Can you work these out from the model? Positions are in its coordinate system, mm. A direction names the side the tool comes from. Coordinates: 2 decimals unless noted, no trailing zeros. Write each loop counter-clockwise with the first axis right and the second up, starting at its lowest first coordinate (ties: lowest second). Pieces come first, ordered by that corner, then holes. Notation, with made-up numbers: (-38.5, 30) - (-4.5, 30) arc R26 cw to (-4.5, 61) - close; hole circle Ø2 at (81, 72). An arc over 180 degrees is marked (long way). Use one line per item in the form item = value. Start each with the question number.
(1) If I drill on probe 1 along Y at (x, z) = (4, 0.2); probe 2 along Y at (x, z) = (21, 1); probe 3 along X at (y, z) = (-40, 1), over which ranges is the centre line in solid material (lowest first)? Write a range as from..to.
(2) If we section it at A-A on x = 12: Please give me the cut outline in (y, z).
(3) If we section it at B-B on z = 0.5: Please give me the cut outline in (x, y).
(4) For pin 1 Ø0.7 at (y, z) = (8, 1.5) entering from +X, with a flat end and sliding along its axis, tell me the tip position at first contact or that it passes through.
(5) On a 3-axis mill with a long thin cutter (end or side, diameter ignored), from which of +Z, -Z, +X, -X, +Y, -Y can I reach the whole of each face in a straight line? I mean faces 4 (the face through (11, 5.879, 2)), 5 (the face through (1, -48, 1)). Say none if no direction works.
(6) Thinking about a two-plate mould opening in Y: for faces 1 (the face through (-0.5, -41, 2)), 2 (the face through (0, 45, 1)), 3 (the face through (-21.64, -47.1, 1.52)), which applies, pulls with the +Y half, pulls with the -Y half, needs draft (parallel to the pull), parting line crosses it, or undercut?
```python
from build123d import *

# Parameters (mm, degrees)
CROQUIS1_W              = 45
CROQUIS1_H              = 93
SALIENTE_EXTRUIR1_DEPTH = 3
CROQUIS2_W              = 23
CROQUIS2_H              = 3.3
CORTAR_EXTRUIR1_DEPTH   = 3
CROQUIS3_W              = 23
CROQUIS3_H              = 3.3
CORTAR_EXTRUIR2_DEPTH   = 3
REDONDEO1_R             = 3
REDONDEO2_R             = 0.5


with BuildPart() as part:
    # Croquis1 → Saliente-Extruir1 (new body)
    with BuildSketch(Plane.XY):
        with Locations((0, -1.5)):
            Rectangle(CROQUIS1_W, CROQUIS1_H)
    extrude(amount=SALIENTE_EXTRUIR1_DEPTH)

    # Croquis2 → Cortar-Extruir1 (cut)
    with BuildSketch(Plane.XY.offset(3)):
        with Locations((11, 7.529451896)):
            Rectangle(CROQUIS2_W, CROQUIS2_H)
    extrude(amount=-CORTAR_EXTRUIR1_DEPTH, mode=Mode.SUBTRACT)

    # Croquis3 → Cortar-Extruir2 (cut)
    with BuildSketch(Plane.XY.offset(3)):
        with Locations((11, -41.35)):
            Rectangle(CROQUIS3_W, CROQUIS3_H)
    extrude(amount=-CORTAR_EXTRUIR2_DEPTH, mode=Mode.SUBTRACT)

    # Redondeo1
    redondeo1_edges = [part.edges().sort_by_distance(p)[0] for p in [
        (-22.5, 45, 1.5),
        (-22.5, -48, 1.5),
        (22.5, 45, 1.5),
    ]]
    fillet(redondeo1_edges, radius=REDONDEO1_R)

    # Redondeo2
    redondeo2_edges = [part.edges().sort_by_distance(p)[0] for p in [
        (-0.5, 9.179451896, 1.5),
        (-0.5, 5.879451896, 1.5),
        (22.5, 5.879451896, 1.5),
        (22.5, 9.179451896, 1.5),
        (-0.5, -39.7, 1.5),
        (-0.5, -43, 1.5),
        (22.5, -43, 1.5),
        (22.5, -39.7, 1.5),
        (22.5, -48, 1.5),
    ]]
    fillet(redondeo2_edges, radius=REDONDEO2_R)


solid = part.part
```
Reported:
q1.probe_1 = -48..-43, -39.7..5.88, 9.18..45
q1.probe_2 = -48..-43, -39.7..5.88, 9.18..44.6
q1.probe_3 = -22.5..-0.46
q2.outline = (-48, 0) - (-43, 0) - (-43, 3) - (-48, 3) - close; (-39.7, 0) - (5.88, 0) - (5.88, 3) - (-39.7, 3) - close; (9.18, 0) - (45, 0) - (45, 3) - (9.18, 3) - close
q3.outline = (-22.5, -45) arc R3 ccw to (-19.5, -48) - (22, -48) arc R0.5 ccw to (22.5, -47.5) - (22.5, -43.5) arc R0.5 ccw to (22, -43) - (0, -43) arc R0.5 cw to (-0.5, -42.5) - (-0.5, -40.2) arc R0.5 cw to (0, -39.7) - (22, -39.7) arc R0.5 ccw to (22.5, -39.2) - (22.5, 5.38) arc R0.5 ccw to (22, 5.88) - (0, 5.88) arc R0.5 cw to (-0.5, 6.38) - (-0.5, 8.68) arc R0.5 cw to (0, 9.18) - (22, 9.18) arc R0.5 ccw to (22.5, 9.68) - (22.5, 42) arc R3 ccw to (19.5, 45) - (-19.5, 45) arc R3 ccw to (-22.5, 42) - close
q4.pin_1 = -0.5
q5.face_4 = +Z, -Z, +X
q5.face_5 = +Z, -Z, +X, -X, -Y
q6.face_1 = undercut
q6.face_2 = pulls with the +Y half
q6.face_3 = pulls with the -Y half
